The model under review builds one solid part; all positions refer to its coordinate system, in mm. Coordinates: 2 decimals unless noted, no trailing zeros. Order: outer loops, then holes, each group sorted by start corner. A loop starts at its lowest first (then second) coordinate and runs counter-clockwise, first axis right, second up. Notation, with made-up numbers: M -15,-2 L 43,-2 A17 ccw 43,13 Z; hole C -34.5,64.25 d11. An arc over 180 degrees is marked long. Answer in a Markdown table with one row per item.
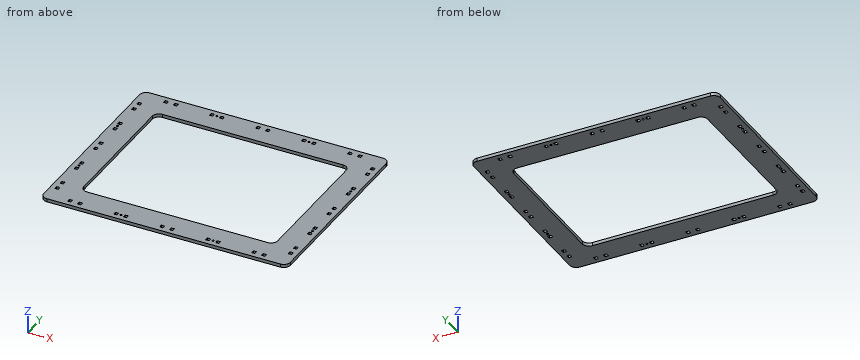
from build123d import *

# Parameters (mm, degrees)
SKETCH1_W           = 375
SKETCH1_H           = 300
SKETCH1_R           = 1.5
SKETCH1_W_2         = 5
SKETCH1_H_2         = 5
BOSS_EXTRUDE2_DEPTH = 5
FILLET1_R           = 10


with BuildPart() as part:
    # Sketch1 → Boss-Extrude2 (new body)
    with BuildSketch(Plane.XY):
        Rectangle(SKETCH1_W, SKETCH1_H)
        with Locations((-177.5, 56)):
            Circle(SKETCH1_R, mode=Mode.SUBTRACT)
        with Locations(Location((177.5, 56, 0), (0, 0, 180))):
            Circle(SKETCH1_R, mode=Mode.SUBTRACT)
        with Locations((-70, 140)):
            Circle(SKETCH1_R, mode=Mode.SUBTRACT)
        with Locations((70, 140)):
            Circle(SKETCH1_R, mode=Mode.SUBTRACT)
        with Locations(Location((70, -140, 0), (0, 0, 180))):
            Circle(SKETCH1_R, mode=Mode.SUBTRACT)
        with Locations(Location((-70, -140, 0), (0, 0, 180))):
            Circle(SKETCH1_R, mode=Mode.SUBTRACT)
        with Locations((177.5, -56)):
            Circle(SKETCH1_R, mode=Mode.SUBTRACT)
        with Locations((-177.5, -56)):
            Circle(SKETCH1_R, mode=Mode.SUBTRACT)
        with Locations((-177.5, -7.5)):
            Rectangle(SKETCH1_W_2, SKETCH1_H_2, mode=Mode.SUBTRACT)
        with Locations((-177.5, 7.5)):
            Rectangle(SKETCH1_W_2, SKETCH1_H_2, mode=Mode.SUBTRACT)
        with Locations((177.5, -63.5)):
            Rectangle(SKETCH1_W_2, SKETCH1_H_2, mode=Mode.SUBTRACT)
        with Locations((-177.5, 104.5)):
            Rectangle(SKETCH1_W_2, SKETCH1_H_2, mode=Mode.SUBTRACT)
        with Locations((-177.5, 119.5)):
            Rectangle(SKETCH1_W_2, SKETCH1_H_2, mode=Mode.SUBTRACT)
        with Locations((-177.5, 48.5)):
            Rectangle(SKETCH1_W_2, SKETCH1_H_2, mode=Mode.SUBTRACT)
        with Locations((-177.5, 63.5)):
            Rectangle(SKETCH1_W_2, SKETCH1_H_2, mode=Mode.SUBTRACT)
        with Locations((177.5, -48.5)):
            Rectangle(SKETCH1_W_2, SKETCH1_H_2, mode=Mode.SUBTRACT)
        with Locations((177.5, 63.5)):
            Rectangle(SKETCH1_W_2, SKETCH1_H_2, mode=Mode.SUBTRACT)
        with Locations((177.5, 48.5)):
            Rectangle(SKETCH1_W_2, SKETCH1_H_2, mode=Mode.SUBTRACT)
        with Locations((177.5, 119.5)):
            Rectangle(SKETCH1_W_2, SKETCH1_H_2, mode=Mode.SUBTRACT)
        with Locations((177.5, 104.5)):
            Rectangle(SKETCH1_W_2, SKETCH1_H_2, mode=Mode.SUBTRACT)
        with Locations((177.5, 7.5)):
            Rectangle(SKETCH1_W_2, SKETCH1_H_2, mode=Mode.SUBTRACT)
        with Locations((177.5, -7.5)):
            Rectangle(SKETCH1_W_2, SKETCH1_H_2, mode=Mode.SUBTRACT)
        with Locations((-147.5, 140)):
            Rectangle(SKETCH1_W_2, SKETCH1_H_2, mode=Mode.SUBTRACT)
        with Locations((-132.5, 140)):
            Rectangle(SKETCH1_W_2, SKETCH1_H_2, mode=Mode.SUBTRACT)
        with Locations((-77.5, 140)):
            Rectangle(SKETCH1_W_2, SKETCH1_H_2, mode=Mode.SUBTRACT)
        with Locations((-62.5, 140)):
            Rectangle(SKETCH1_W_2, SKETCH1_H_2, mode=Mode.SUBTRACT)
        with Locations((-7.5, 140)):
            Rectangle(SKETCH1_W_2, SKETCH1_H_2, mode=Mode.SUBTRACT)
        with Locations((7.5, 140)):
            Rectangle(SKETCH1_W_2, SKETCH1_H_2, mode=Mode.SUBTRACT)
        with Locations((62.5, 140)):
            Rectangle(SKETCH1_W_2, SKETCH1_H_2, mode=Mode.SUBTRACT)
        with Locations((77.5, 140)):
            Rectangle(SKETCH1_W_2, SKETCH1_H_2, mode=Mode.SUBTRACT)
        with Locations((132.5, 140)):
            Rectangle(SKETCH1_W_2, SKETCH1_H_2, mode=Mode.SUBTRACT)
        with Locations((147.5, 140)):
            Rectangle(SKETCH1_W_2, SKETCH1_H_2, mode=Mode.SUBTRACT)
        with Locations((147.5, -140)):
            Rectangle(SKETCH1_W_2, SKETCH1_H_2, mode=Mode.SUBTRACT)
        with Locations((132.5, -140)):
            Rectangle(SKETCH1_W_2, SKETCH1_H_2, mode=Mode.SUBTRACT)
        with Locations((77.5, -140)):
            Rectangle(SKETCH1_W_2, SKETCH1_H_2, mode=Mode.SUBTRACT)
        with Locations((62.5, -140)):
            Rectangle(SKETCH1_W_2, SKETCH1_H_2, mode=Mode.SUBTRACT)
        with Locations((7.5, -140)):
            Rectangle(SKETCH1_W_2, SKETCH1_H_2, mode=Mode.SUBTRACT)
        with Locations((-7.5, -140)):
            Rectangle(SKETCH1_W_2, SKETCH1_H_2, mode=Mode.SUBTRACT)
        with Locations((-62.5, -140)):
            Rectangle(SKETCH1_W_2, SKETCH1_H_2, mode=Mode.SUBTRACT)
        with Locations((-77.5, -140)):
            Rectangle(SKETCH1_W_2, SKETCH1_H_2, mode=Mode.SUBTRACT)
        with Locations((-132.5, -140)):
            Rectangle(SKETCH1_W_2, SKETCH1_H_2, mode=Mode.SUBTRACT)
        with Locations((-147.5, -140)):
            Rectangle(SKETCH1_W_2, SKETCH1_H_2, mode=Mode.SUBTRACT)
        with BuildLine():
            Line((-137.5, -110), (137.5, -110))
            ThreePointArc((137.5, -110), (144.571067812, -107.071067812), (147.5, -100))
            Line((147.5, -100), (147.5, 100))
            ThreePointArc((147.5, 100), (144.571067812, 107.071067812), (137.5, 110))
            Line((137.5, 110), (-137.5, 110))
            ThreePointArc((-137.5, 110), (-144.571067812, 107.071067812), (-147.5, 100))
            Line((-147.5, 100), (-147.5, -100))
            ThreePointArc((-147.5, -100), (-144.571067812, -107.071067812), (-137.5, -110))
        make_face(mode=Mode.SUBTRACT)
        with Locations((177.5, -119.5)):
            Rectangle(SKETCH1_W_2, SKETCH1_H_2, mode=Mode.SUBTRACT)
        with Locations((177.5, -104.5)):
            Rectangle(SKETCH1_W_2, SKETCH1_H_2, mode=Mode.SUBTRACT)
        with Locations((-177.5, -119.5)):
            Rectangle(SKETCH1_W_2, SKETCH1_H_2, mode=Mode.SUBTRACT)
        with Locations((-177.5, -104.5)):
            Rectangle(SKETCH1_W_2, SKETCH1_H_2, mode=Mode.SUBTRACT)
        with Locations((-177.5, -63.5)):
            Rectangle(SKETCH1_W_2, SKETCH1_H_2, mode=Mode.SUBTRACT)
        with Locations((-177.5, -48.5)):
            Rectangle(SKETCH1_W_2, SKETCH1_H_2, mode=Mode.SUBTRACT)
    extrude(amount=BOSS_EXTRUDE2_DEPTH)

    # Fillet1
    fillet1_edges = [part.edges().sort_by_distance(p)[0] for p in [
        (187.5, -150, 2.5),
        (-187.5, -150, 2.5),
        (-187.5, 150, 2.5),
        (187.5, 150, 2.5),
    ]]
    fillet(fillet1_edges, radius=FILLET1_R)


solid = part.part
(1) Insertion check: P1, Ø2.5, axis at y = 140.5, z = 2.5, coming from the +X side; P2, Ø1, axis at x = -145.5, y = 1, coming from the +Z side. Each pin has a flat end and moves straight along its axis. Give the tip position at first contact, or say it passes through.
Report:
| item | result |
|---|---|
| P1 | x = 187.5 |
| P2 | through |
(2) To check wall thickness, follow line 1 (X direction, y = 118.5, z = 3.55); line 2 (Y direction, x = -70, z = 3.85); line 3 (X direction, y = 47, z = 0.35). State the ranges of each line that lie inside material, in increasing order. Write a range as [from, to].
Report:
| item | result |
|---|---|
| line 1 | [-187.5, -180], [-175, 175], [180, 187.5] |
| line 2 | [-150, -141.5], [-138.5, -110], [110, 138.5], [141.5, 150] |
| line 3 | [-187.5, -180], [-175, -147.5], [147.5, 175], [180, 187.5] |
(3) Take a section at B-B (x = 31.5). Write out the cut boundary in (y, z), then the cut area to 3 significant figures.
Report:
| item | result |
|---|---|
| outline | M -150,0 L -110,0 L -110,5 L -150,5 Z; M 110,0 L 150,0 L 150,5 L 110,5 Z |
| area | 400 mm^2 |
(4) Take a section at C-C (z = 3.25). State how many separate pieces and enclosed holes the cut face has, then the cut area to 3 significant figures.
Report:
| item | result |
|---|---|
| separate pieces | 1 |
| enclosed holes | 49 |
| area | 46,500 mm^2 |
(5) Take a section at A-A (y = -34.5). Write out the cut boundary in (x, z).
Report:
| item | result |
|---|---|
| outline | M -187.5,0 L -147.5,0 L -147.5,5 L -187.5,5 Z; M 147.5,0 L 187.5,0 L 187.5,5 L 147.5,5 Z |
